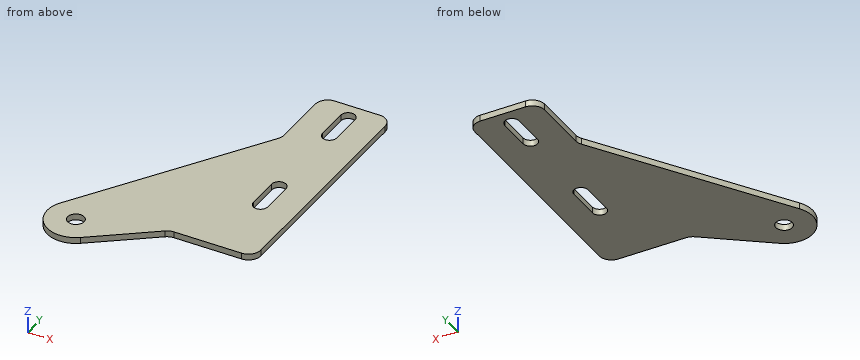
from build123d import *

# Parameters (mm, degrees)
ESQUISSE1_R               = 2
T_LE_DE_BASE_PLI_E1_DEPTH = 1.5
CONG_1_R                  = 3


# Sheet-metal steps are written as plain solids
with BuildPart() as part:
    # Esquisse1 → Tôle de base pliée1 (new body)
    with BuildSketch(Plane.XY):
        with BuildLine():
            Line((-27.270863059, -33.578028391), (-12, -22))
            Line((-12, -22), (8.5, -22))
            Line((8.5, -22), (8.5, 38))
            Line((8.5, 38), (-8.5, 38))
            Line((-8.5, 38), (-8.5, 20.557195103))
            Line((-8.5, 20.557195103), (-37.381886846, -24.204817905))
            ThreePointArc((-37.381886846, -24.204817905), (-36.258903683, -33.133501313), (-27.270863059, -33.578028391))
        make_face()
        with Locations((-31.5, -28)):
            Circle(ESQUISSE1_R, mode=Mode.SUBTRACT)
        with BuildLine():
            Line((1.75, 4), (1.75, -4))
            ThreePointArc((1.75, -4), (0, -5.75), (-1.75, -4))
            Line((-1.75, -4), (-1.75, 4))
            ThreePointArc((-1.75, 4), (0, 5.75), (1.75, 4))
        make_face(mode=Mode.SUBTRACT)
        with BuildLine():
            Line((1.75, 34), (1.75, 26))
            ThreePointArc((1.75, 26), (0, 24.25), (-1.75, 26))
            Line((-1.75, 26), (-1.75, 34))
            ThreePointArc((-1.75, 34), (0, 35.75), (1.75, 34))
        make_face(mode=Mode.SUBTRACT)
    extrude(amount=-T_LE_DE_BASE_PLI_E1_DEPTH)

    # Congé1
    cong_1_edges = [part.edges().sort_by_distance(p)[0] for p in [
        (-8.5, 38, -0.75),
        (8.5, 38, -0.75),
        (8.5, -22, -0.75),
        (-12, -22, -0.75),
        (-8.5, 20.557195103, -0.75),
    ]]
    fillet(cong_1_edges, radius=CONG_1_R)


solid = part.part
Geometry check sheet. Reference: the model listing, model coordinates, mm. Give positions to 0.01 mm unless a question says otherwise; leave off trailing zeros. Write each loop counter-clockwise with the first axis right and the second up, starting at its lowest first coordinate (ties: lowest second). Pieces come first, ordered by that corner, then holes.
1) Cross-section at B-B (x = 0). Record the boundary of the cut face in (y, z), plus the area to 3 significant figures.
Values follow:
outline: (-22, -1.5) - (-5.75, -1.5) - (-5.75, 0) - (-22, 0) - close; (5.75, -1.5) - (24.25, -1.5) - (24.25, 0) - (5.75, 0) - close; (35.75, -1.5) - (38, -1.5) - (38, 0) - (35.75, 0) - close
area: 55.5 mm2
2) Cross-section at A-A (z = -0.95). Record the boundary of the cut face in (x, y), plus the area to 3 significant figures.
Values follow:
outline: (-37.38, -24.2) arc R7 ccw to (-27.27, -33.58) - (-12.8, -22.61) arc R3 cw to (-10.99, -22) - (5.5, -22) arc R3 ccw to (8.5, -19) - (8.5, 35) arc R3 ccw to (5.5, 38) - (-5.5, 38) arc R3 ccw to (-8.5, 35) - (-8.5, 21.44) arc R3 cw to (-8.98, 19.81) - close; hole circle Ø4 at (-31.5, -28); hole (-1.75, -4) arc R1.75 ccw to (1.75, -4) - (1.75, 4) arc R1.75 ccw to (-1.75, 4) - close; hole (-1.75, 26) arc R1.75 ccw to (1.75, 26) - (1.75, 34) arc R1.75 ccw to (-1.75, 34) - close
area: 1,730 mm2
3) Cross-section at D-D (x = -31.5). Record the boundary of the cut face in (y, z).
Values follow:
outline: (-35, -1.5) - (-30, -1.5) - (-30, 0) - (-35, 0) - close; (-26, -1.5) - (-15.09, -1.5) - (-15.09, 0) - (-26, 0) - close
4) Go/stop test with flat-tipped pins: pin 1 Ø0.8 at (y, z) = (0, -0.5) entering from -X; pin 2 Ø0.8 at (x, z) = (-5.5, -1) entering from -Y. Record where each tip stops, or that it passes through.
Values follow:
pin 1: stops at x = -22.02
pin 2: stops at y = -22
5) Cross-section at C-C (y = 32). Record the boundary of the cut face in (x, z), plus the area to 4 significant figures.
Values follow:
outline: (-8.5, -1.5) - (-1.75, -1.5) - (-1.75, 0) - (-8.5, 0) - close; (1.75, -1.5) - (8.5, -1.5) - (8.5, 0) - (1.75, 0) - close
area: 20.25 mm2
6) Thickness scan on line 1 (Y direction, x = 1.5, z = -0.2); line 2 (X direction, y = 33, z = -1.1); line 3 (Y direction, x = -31.5, z = -0.75). Record the ranges inside material, lowest first.
Values follow:
line 1: y = -22 to -4.9, 4.9 to 25.1, 34.9 to 38
line 2: x = -8.5 to -1.75, 1.75 to 8.5
line 3: y = -35 to -30, -26 to -15.09
